```python
from build123d import *

# Parameters (mm, degrees)
SKETCH1_R           = 2.032
BOSS_EXTRUDE4_DEPTH = 5.08


with BuildPart() as part:
    # Sketch1 → Boss-Extrude4 (new body)
    with BuildSketch(Plane(origin=(0, 0, 0), x_dir=(1, 0, 0), z_dir=(0, 1, 0))):
        Polygon((38.1, -82.48891971), (47.625, -82.48891971), (95.25, 0), (90.4875, 8.248891971), (79.488977372, 1.898891971), (41.388977372, 67.890027739), (52.3875, 74.240027739), (47.625, 82.48891971), (-47.625, 82.48891971), (-52.3875, 74.240027739), (-41.388977372, 67.890027739), (-79.488977372, 1.898891971), (-90.4875, 8.248891971), (-95.25, 0), (-47.625, -82.48891971), (-38.1, -82.48891971), (-38.1, -69.78891971), (38.1, -69.78891971), align=None)
        with Locations(Location((-50.913977372, -51.392243797, 0), (0, 0, 270))):
            Circle(SKETCH1_R, mode=Mode.SUBTRACT)
        with Locations(Location((-15.875, -63.43891971, 0), (0, 0, 270))):
            Circle(SKETCH1_R, mode=Mode.SUBTRACT)
        with Locations(Location((-69.963977372, -18.396675913, 0), (0, 0, 270))):
            Circle(SKETCH1_R, mode=Mode.SUBTRACT)
        with Locations(Location((15.875, -63.43891971, 0), (0, 0, 270))):
            Circle(SKETCH1_R, mode=Mode.SUBTRACT)
        with Locations(Location((50.913977372, -51.392243797, 0), (0, 0, 270))):
            Circle(SKETCH1_R, mode=Mode.SUBTRACT)
        with Locations(Location((69.963977372, -18.396675913, 0), (0, 0, 270))):
            Circle(SKETCH1_R, mode=Mode.SUBTRACT)
        with Locations(Location((-62.877216058, 17.97130657, 0), (0, 0, 270))):
            Circle(SKETCH1_R, mode=Mode.SUBTRACT)
        with Locations(Location((-47.002216058, 45.46761314, 0), (0, 0, 270))):
            Circle(SKETCH1_R, mode=Mode.SUBTRACT)
        with Locations(Location((-19.05, 69.78891971, 0), (0, 0, 270))):
            Circle(SKETCH1_R, mode=Mode.SUBTRACT)
        with Locations(Location((62.877216058, 17.97130657, 0), (0, 0, 270))):
            Circle(SKETCH1_R, mode=Mode.SUBTRACT)
        with Locations(Location((47.002216058, 45.46761314, 0), (0, 0, 270))):
            Circle(SKETCH1_R, mode=Mode.SUBTRACT)
        with Locations(Location((19.05, 69.78891971, 0), (0, 0, 270))):
            Circle(SKETCH1_R, mode=Mode.SUBTRACT)
    extrude(amount=BOSS_EXTRUDE4_DEPTH)


solid = part.part
```
Verification items for the finished model (mm, model axes). A direction names the side the tool comes from. Give positions to 0.01 mm unless a question says otherwise; leave off trailing zeros. Loops run counter-clockwise (first coordinate to the right, second up) from the corner with the lowest first, then second, coordinate; pieces in that order, holes last.
1. Go/stop test with flat-tipped pins: pin 1 Ø3.5 at (x, z) = (15.88, 63.44) entering from -Y; pin 2 Ø3 at (x, y) = (-71, 4) entering from +Z; pin 3 Ø2.5 at (x, y) = (-14, 2) entering from +Z. Record where each tip stops, or that it passes through.
2. Section check B-B, the plane x = -77. Enter the section's corners in (y, z), then the cut area to 3 significant figures.
3. Set-up check for faces 5 (the flat face through (85.07, 2.5, -5.12)), 6 (the flat face through (-92.835, 2.504, -4.182)), 7 (the flat face through (-38.1, 3, 76)): record each of +Z, -Z, +X, -X, +Y, -Y from which the full face is reachable in a straight line by a thin tool's end or side.
4. Section check C-C, the plane z = 45. Enter the section's corners in (x, y).
5. Section check A-A, the plane z = -4.5. Enter the section's corners in (x, y), then the cut area to 3 significant figures.
6. Thickness scan on line 1 (X direction, y = 3.25, z = -5); line 2 (Z direction, x = -24, y = 1.8); line 3 (X direction, y = 2.95, z = -71). Record the ranges inside material, lowest first.
7. Mould release check, pull along X, two halves, no side actions. Record for faces 1 (the flat face through (-84.91, 2.5, -5.03)), 2 (the flat face through (1, 3, -82.489)), 3 (the cylindrical face through (-47.8, 2.5, -43.6)), 4 (the flat face through (50.04, 2.5, -78.31)): released by +X, released by -X, zero draft, split by the parting line, or undercut.
Geometry says:
1. pin 1: passes through
1. pin 2: stops at z = 44.6
1. pin 3: stops at z = 69.79
2. outline: (0, -6.21) - (5.08, -6.21) - (5.08, 31.61) - (0, 31.61) - close
2. area: 192 mm2
3. face 5: -Z, +Y, -Y
3. face 6: -Z, -X, +Y, -Y
3. face 7: +Z, +Y, -Y
4. outline: (-69.27, 0) - (69.27, 0) - (69.27, 5.08) - (-69.27, 5.08) - close
5. outline: (-92.65, 0) - (-83.99, 0) - (-83.99, 5.08) - (-92.65, 5.08) - close; (-77.99, 0) - (77.99, 0) - (77.99, 5.08) - (-77.99, 5.08) - close; (83.99, 0) - (92.65, 0) - (92.65, 5.08) - (83.99, 5.08) - close
5. area: 880 mm2
6. line 1: x = -92.36 to -84.86, -77.7 to 77.7, 84.86 to 92.36
6. line 2: z = -82.49 to 69.79
6. line 3: x = -46.78 to -20.68, -17.42 to 17.42, 20.68 to 46.78
7. face 1: undercut
7. face 2: zero draft
7. face 3: undercut
7. face 4: released by +X
